from build123d import *

# Parameters (mm, degrees)
BOSS_EXTRUDE1_DEPTH  = 8
CUT_EXTRUDE1_DEPTH   = 9
M3_CLEARANCE_HOLE1_D = 3.4
FILLET1_R            = 0.5


with BuildPart() as part:
    # Sketch1 → Boss-Extrude1 (new body)
    with BuildSketch(Plane(origin=(0, 8, 0), x_dir=(1, 0, 0), z_dir=(0, 1, 0))):
        Polygon((34.769686411, 2), (20.35, 4), (14.35, 4), (-0.069686411, 2), (0, 0), (14.35, 0.5), (20.35, 0.5), (34.7, 0), align=None)
    extrude(amount=-BOSS_EXTRUDE1_DEPTH)

    # Sketch2 → Cut-Extrude1 (cut, through all)
    with BuildSketch(Plane.XZ):
        with BuildLine():
            Line((5.968779898, -1.482280416), (14.35, -2.5))
            Line((14.35, -2.5), (20.35, -2.5))
            Line((20.35, -2.5), (28.731220102, -1.482280416))
            ThreePointArc((28.731220102, -1.482280416), (28.818634048, -1.372710787), (28.710625676, -1.283374942))
            Line((28.710625676, -1.283374942), (20.35, -2))
            Line((20.35, -2), (14.35, -2))
            Line((14.35, -2), (5.989374324, -1.283374942))
            ThreePointArc((5.989374324, -1.283374942), (5.881365952, -1.372710787), (5.968779898, -1.482280416))
        make_face()
    extrude(amount=-CUT_EXTRUDE1_DEPTH, mode=Mode.SUBTRACT)

    # M3 Clearance Hole1 (through all)
    with Locations(Plane.XY.offset(-0.5)):
        with Locations((17.35, 4)):
            Hole(M3_CLEARANCE_HOLE1_D / 2)

    # Fillet1
    fillet1_edges = [part.edges().sort_by_distance(p)[0] for p in [
        (34.7, 4, 0),
        (0, 4, 0),
        (-0.069686411, 4, -2),
        (34.769686411, 4, -2),
    ]]
    fillet(fillet1_edges, radius=FILLET1_R)


solid = part.part
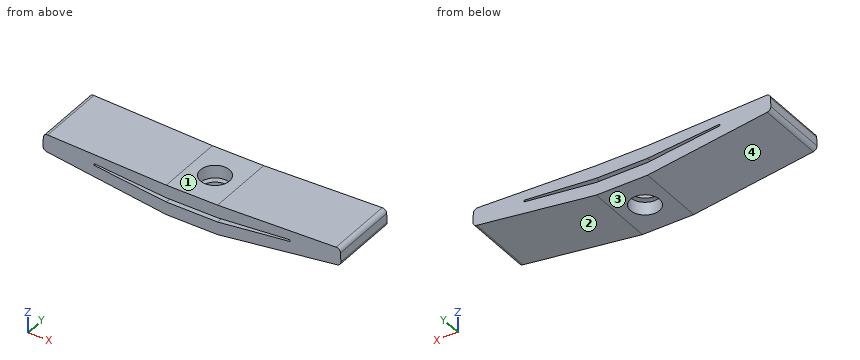
Can you work these out from the model? Positions are in its coordinate system, mm. Face numbers are marked on the shaded views. Give positions to 0.01 mm unless a question says otherwise; leave off trailing zeros. Write each loop counter-clockwise with the first axis right and the second up, starting at its lowest first coordinate (ties: lowest second). Pieces come first, ordered by that corner, then holes. Notation, with made-up numbers: (42.5, 86) -> (88.5, 86) arc R30 cw to (88.5, 109) -> close; hole circle Ø4 at (15, -19.75). An arc over 180 degrees is marked (long way). Answer as a JSON object with one key per item and string values. Group by question number.
Item 1: Please list where these lines run through material, in increasing order: line 1 (Y direction, x = 17.35, z = -1.6); line 2 (Z direction, x = 27.5, y = 6); line 3 (Z direction, x = 11.5, y = 4.25). Write a range as [from, to].
Item 2: Suppose I cut it at B-B (x = 17.35). Please give me the cut outline in (y, z), plus the area to 3 significant figures.
Item 3: Suppose I cut it at D-D (x = 21). Please give me the cut outline in (y, z).
Item 4: We'd pull the mould along X, two halves only. Please class the marked faces 1, 2, 3 and 4: +X half, -X half, draft (parallel to the pull), parting line (faces both ways), or undercut.
Item 5: Suppose I cut it at A-A (y = 4). Please give me the cut outline in (x, z).
Item 6: Suppose I cut it at C-C (y = 1.5). Please give me the cut outline in (x, z), plus the area to 3 significant figures.
Item 7: I'm going to push flat-ended pins straight in: P1, Ø1, axis at x = 7, y = 6, coming from the -Z side; P2, Ø3, axis at x = 17.5, y = 2.5, coming from the +Z side; P3, Ø3, axis at x = 17.35, y = 4, coming from the +Z side. Where does each tip first touch, or does it pass through?
Findings:
{
 "1": {"line 1": "y = [0, 2.3], [5.7, 8]", "line 2": "z = [-3.01, -1.63], [-1.39, -0.25]", "line 3": "z = [-3.6, -2.15], [-1.76, -0.4]"},
 "2": {"outline": "(0, -4) -> (2.3, -4) -> (2.3, -2.5) -> (0, -2.5) -> close; (0, -2) -> (2.3, -2) -> (2.3, -0.5) -> (0, -0.5) -> close; (5.7, -4) -> (8, -4) -> (8, -2.5) -> (5.7, -2.5) -> close; (5.7, -2) -> (8, -2) -> (8, -0.5) -> (5.7, -0.5) -> close", "area": "13.8 mm²"},
 "3": {"outline": "(0, -3.91) -> (8, -3.91) -> (8, -2.42) -> (0, -2.42) -> close; (0, -1.94) -> (8, -1.94) -> (8, -0.48) -> (0, -0.48) -> close"},
 "4": {"face 1": "undercut", "face 2": "+X half", "face 3": "draft", "face 4": "-X half"},
 "5": {"outline": "(-0.05, -1.55) arc R0.5 ccw to (0.38, -2.06) -> (14.35, -4) -> (15.65, -4) -> (15.65, -2.5) -> (14.35, -2.5) -> (5.97, -1.48) arc R0.1 cw to (5.99, -1.28) -> (14.35, -2) -> (15.65, -2) -> (15.65, -0.5) -> (14.35, -0.5) -> (0.5, -0.02) arc R0.5 ccw to (-0.02, -0.5) -> close; (19.05, -4) -> (20.35, -4) -> (34.32, -2.06) arc R0.5 ccw to (34.75, -1.55) -> (34.72, -0.5) arc R0.5 ccw to (34.2, -0.02) -> (20.35, -0.5) -> (19.05, -0.5) -> (19.05, -2) -> (20.35, -2) -> (28.71, -1.28) arc R0.1 cw to (28.73, -1.48) -> (20.35, -2.5) -> (19.05, -2.5) -> close"},
 "6": {"outline": "(-0.05, -1.55) arc R0.5 ccw to (0.38, -2.06) -> (14.35, -4) -> (20.35, -4) -> (34.32, -2.06) arc R0.5 ccw to (34.75, -1.55) -> (34.72, -0.5) arc R0.5 ccw to (34.2, -0.02) -> (20.35, -0.5) -> (14.35, -0.5) -> (0.5, -0.02) arc R0.5 ccw to (-0.02, -0.5) -> close; hole (5.97, -1.48) -> (14.35, -2.5) -> (20.35, -2.5) -> (28.73, -1.48) arc R0.1 ccw to (28.71, -1.28) -> (20.35, -2) -> (14.35, -2) -> (5.99, -1.28) arc R0.1 ccw to start", "area": "91.1 mm²"},
 "7": {"P1": "stops at z = -3.05", "P2": "stops at z = -0.5", "P3": "passes through"}
}
